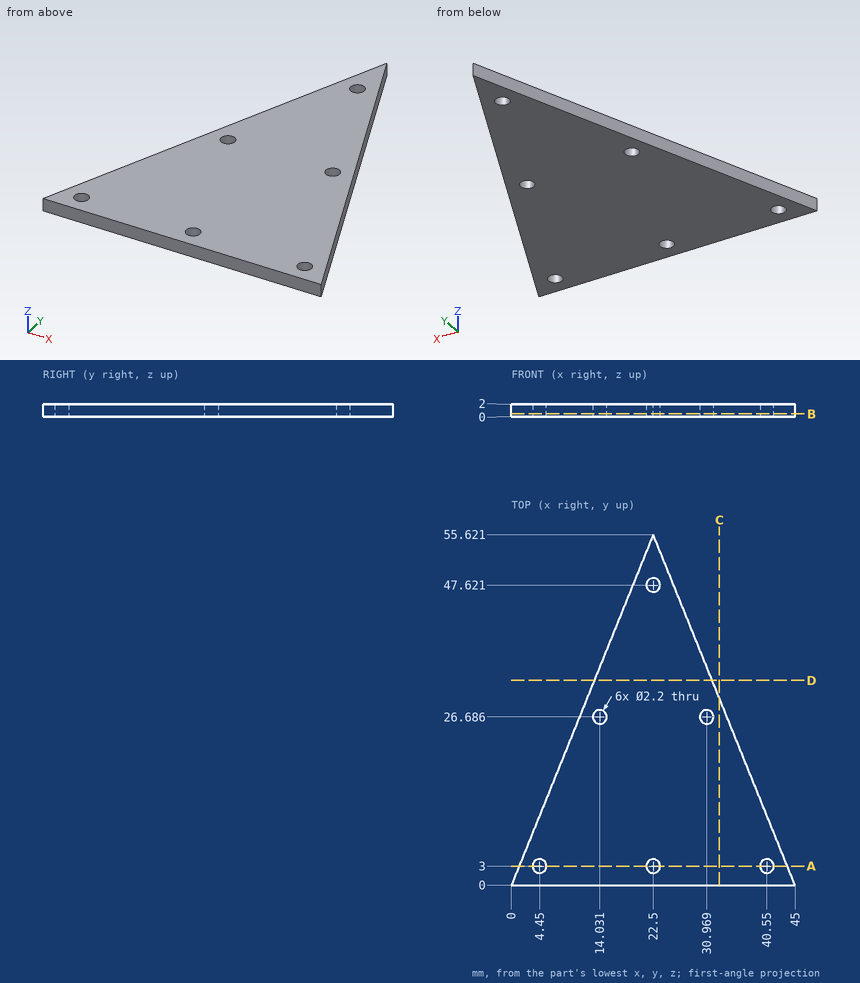
Design review of the part shown in the three views and the two pictorial views. Dimensions are in mm from the part's minimum x, y and z. Round coordinates to 2 decimals unless told otherwise and drop trailing zeros. Write each loop counter-clockwise with the first axis right and the second up, starting at its lowest first coordinate (ties: lowest second). Pieces come first, ordered by that corner, then holes.
Item 1: Wall thickness on L1, parallel to X at y = 26.5, z = 0.55 (1 decimal); L2, parallel to Y at x = 23, z = 0.8 (1 decimal); L3, parallel to Y at x = 14, z = 1.6 (1 decimal): over which ranges is each line inside the solid? List them lowest first.
Item 2: Consider section C-C on x = 33. Give the boundary of the cut face in (y, z) (1 decimal).
Item 3: Consider section A-A on y = 3. Give the boundary of the cut face in (x, z).
Item 4: Consider section D-D on y = 32.5. Give the boundary of the cut face in (x, z).
Item 5: Consider section B-B on z = 0.45. Count the separate pieces of the cut face and the enclosed holes in it, and give its area (3 significant figures).
Check values:
1. L1: x = 10.7 to 12.9, 15.1 to 29.9, 32.1 to 34.3
1. L2: y = 0 to 2, 4 to 46.6, 48.6 to 54.4
1. L3: y = 0 to 25.6, 27.8 to 34.6
2. outline: (0, 0) - (29.7, 0) - (29.7, 2) - (0, 2) - close
3. outline: (1.21, 0) - (3.35, 0) - (3.35, 2) - (1.21, 2) - close; (5.55, 0) - (21.4, 0) - (21.4, 2) - (5.55, 2) - close; (23.6, 0) - (39.45, 0) - (39.45, 2) - (23.6, 2) - close; (41.65, 0) - (43.79, 0) - (43.79, 2) - (41.65, 2) - close
4. outline: (13.15, 0) - (31.85, 0) - (31.85, 2) - (13.15, 2) - close
5. separate pieces: 1
5. enclosed holes: 6
5. area: 1,230 mm2
